The model under review builds one solid part; all positions refer to its coordinate system, in mm. Face numbers are marked on the shaded views. A direction names the side the tool comes from. Coordinates: 2 decimals unless noted, no trailing zeros. Order: outer loops, then holes, each group sorted by start corner. A loop starts at its lowest first (then second) coordinate and runs counter-clockwise, first axis right, second up. Notation, with made-up numbers: M 13.5,-2.75 L 41.5,-2.75 A22 cw 41.5,21.25 Z; hole C 10.5,39.5 d6. An arc over 180 degrees is marked long. One line per item, written item: value.
```python
from build123d import *

# Parameters (mm, degrees)
CROQUIS1_R              = 2.1
SALIENTE_EXTRUIR1_DEPTH = 4
SALIENTE_EXTRUIR2_START = -8
CROQUIS1_5_R            = 2.1
SALIENTE_EXTRUIR2_DEPTH = 8
REDONDEO2_R             = 2
CROQUIS1_6_R            = 2.1
SALIENTE_EXTRUIR3_DEPTH = 15
REDONDEO1_R             = 10


with BuildPart() as part:
    # Croquis1 → Saliente-Extruir1 (new body)
    with BuildSketch(Plane.XY):
        with BuildLine():
            Line((10, 54), (10, -54))
            ThreePointArc((10, -54), (0, -64), (-10, -54))
            Line((-10, -54), (-10, 54))
            ThreePointArc((-10, 54), (0, 64), (10, 54))
        make_face()
        with Locations((0, 54)):
            Circle(CROQUIS1_R, mode=Mode.SUBTRACT)
        with Locations((0, -54)):
            Circle(CROQUIS1_R, mode=Mode.SUBTRACT)
        with BuildLine():
            Line((6, 38), (6, -38))
            ThreePointArc((6, -38), (0, -44), (-6, -38))
            Line((-6, -38), (-6, 38))
            ThreePointArc((-6, 38), (0, 44), (6, 38))
        make_face(mode=Mode.SUBTRACT)
    extrude(amount=SALIENTE_EXTRUIR1_DEPTH)

    # Croquis1<5> → Saliente-Extruir2 (add)
    with BuildSketch(Plane.XY.offset(SALIENTE_EXTRUIR2_START)):
        with BuildLine():
            Line((10, -54), (10, -47.95))
            Line((10, -47.95), (-10, -47.95))
            Line((-10, -47.95), (-10, -54))
            ThreePointArc((-10, -54), (0, -64), (10, -54))
        make_face()
        with Locations((0, -54)):
            Circle(CROQUIS1_5_R, mode=Mode.SUBTRACT)
    extrude(amount=SALIENTE_EXTRUIR2_DEPTH)

    # Redondeo2
    redondeo2_edges = [part.edges().sort_by_distance(p)[0] for p in [
        (0, -47.95, 0),
        (0, -47.95, -8),
    ]]
    fillet(redondeo2_edges, radius=REDONDEO2_R)

    # Croquis1<6> → Saliente-Extruir3 (add)
    with BuildSketch(Plane.XY):
        with BuildLine():
            Line((10, 47.95), (10, 54))
            ThreePointArc((10, 54), (0, 64), (-10, 54))
            Line((-10, 54), (-10, 47.95))
            Line((-10, 47.95), (10, 47.95))
        make_face()
        with Locations((0, 54)):
            Circle(CROQUIS1_6_R, mode=Mode.SUBTRACT)
    extrude(amount=SALIENTE_EXTRUIR3_DEPTH)

    # Redondeo1
    # the kernel refuses this fillet: 10 mm, written as the material it adds along each edge
    with BuildSketch(Plane(origin=(-10, 47.95, 4), x_dir=(0, 0, 1), z_dir=(1, 0, 0))) as redondeo1_piece_1_section:
        with BuildLine():
            CenterArc((REDONDEO1_R, REDONDEO1_R), REDONDEO1_R, 180, 90)
            Line((0, REDONDEO1_R), (0, 0))
            Line((0, 0), (REDONDEO1_R, 0))
        make_face()
    redondeo1_piece_1 = extrude(amount=20, mode=Mode.PRIVATE)
    redondeo1_piece_1 = redondeo1_piece_1 - Plane(origin=(0, 38, 6.263951143), x_dir=(-1, 0, 0), z_dir=(0, 0, -1)) * Cylinder(6, 80, mode=Mode.PRIVATE)
    add(redondeo1_piece_1)


solid = part.part
```
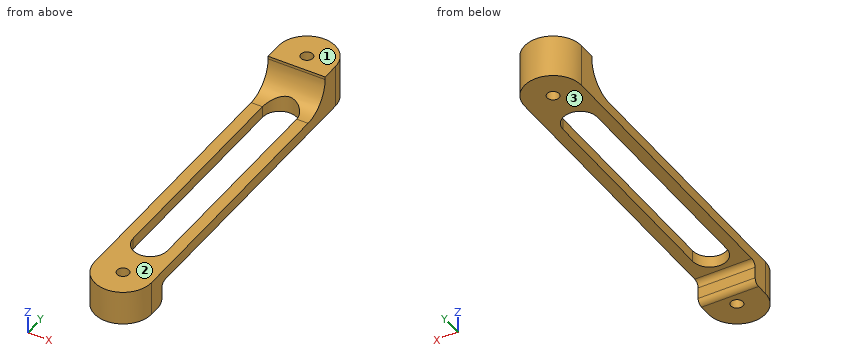
(1) For L1, parallel to Y at x = 0, z = -3.25; L2, parallel to Z at x = -1, y = 58; L3, parallel to Y at x = 0, z = -1.25, list the stretches that pass through material, from the lowest coordinate up.
Geometry results:
L1: y = -64 to -56.1, -51.9 to -47.95
L2: z = 0 to 15
L3: y = -64 to -56.1, -51.9 to -47.8
(2) We need section C-C, the plane x = -7.75. State the section outline as (y, z) points, plus the area to 3 significant figures.
Geometry results:
outline: M -60.32,-8 L -49.95,-8 A2 ccw -47.95,-6 L -47.95,-2 A2 cw -45.95,0 L 60.32,0 L 60.32,15 L 47.95,15 L 47.95,14 A10 cw 37.95,4 L -60.32,4 Z
area: 739 mm2
(3) We need section A-A, the plane x = -1. State the section outline as (y, z) points.
Geometry results:
outline: M -63.95,-8 L -55.85,-8 L -55.85,4 L -63.95,4 Z; M -52.15,-8 L -49.95,-8 A2 ccw -47.95,-6 L -47.95,-2 A2 cw -45.95,0 L -43.92,0 L -43.92,4 L -52.15,4 Z; M 43.92,0 L 52.15,0 L 52.15,15 L 47.95,15 L 47.95,14 A10 cw 43.92,5.97 Z; M 55.85,0 L 63.95,0 L 63.95,15 L 55.85,15 Z
(4) We need section B-B, the plane y = 9.5. State the section outline as (x, z) points.
Geometry results:
outline: M -10,0 L -6,0 L -6,4 L -10,4 Z; M 6,0 L 10,0 L 10,4 L 6,4 Z
(5) Tool access review of the marked faces 1, 2 and 3: name each direction out of +Z, -Z, +X, -X, +Y, -Y from which nothing blocks a thin tool from reaching the whole face with its end or side.
Geometry results:
face 1: +Z, +X, -X, +Y, -Y
face 2: +Z, +X, -X, -Y
face 3: -Z, +X, -X, +Y
(6) Insertion check: pin 1 Ø6.5 at (x, y) = (0, 54) entering from +Z; pin 2 Ø5 at (x, y) = (3.5, 43.5) entering from -Z; pin 3 Ø1.1 at (x, z) = (-0.5, 14.5) entering from -Y; pin 4 Ø10 at (x, y) = (-7.5, -27) entering from +Z. Each pin has a flat end and moves straight along its axis. Give the tip position at first contact, or say it passes through.
Geometry results:
pin 1: stops at z = 15
pin 2: stops at z = 0
pin 3: stops at y = 47.95
pin 4: stops at z = 4
